Verification items for this drawing (mm, ordinates from the low corner). A direction names the side the tool comes from. Round coordinates to 2 decimals unless told otherwise and drop trailing zeros. Order: outer loops, then holes, each group sorted by start corner. A loop starts at its lowest first (then second) coordinate and runs counter-clockwise, first axis right, second up. Notation, with made-up numbers: M -15,-28 L 42,-28 A27 cw 42,-8 Z; hole C 30.25,36.5 d10. An arc over 180 degrees is marked long. Return JSON: item names as keys, results as strings. Group by question number.
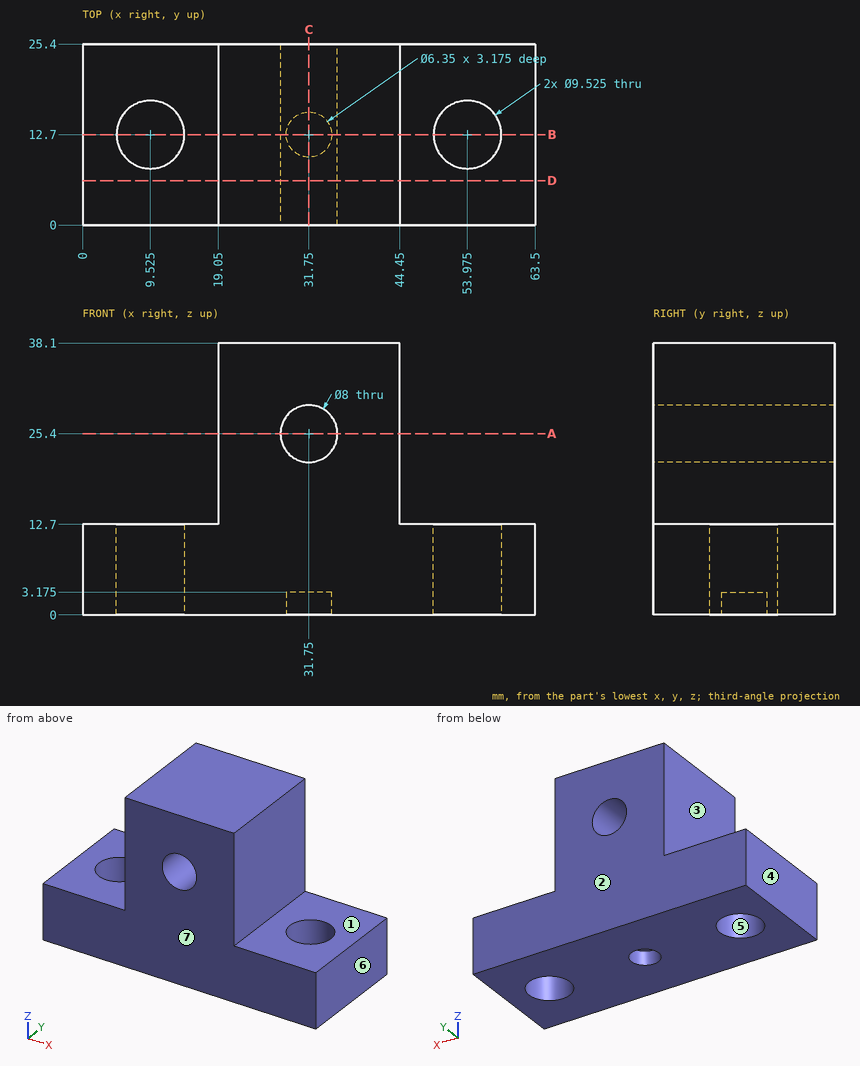
1. Draft check along X on the marked faces 4, 5, 6 and 7. Enter one of: +X half, -X half, draft (parallel to the pull), parting line (faces both ways), or undercut.
2. Cross-section at D-D (y = 6.25). Enter the section's corners in (x, z), plus the area to 3 significant figures.
3. Go/stop test with flat-tipped pins: pin 1 (4 mm diameter, centred on y = 21.5, z = 19.5, fed in from -X); pin 2 (9.5 mm diameter, centred on x = 11.5, y = 17.5, fed in from +Z); pin 3 (5 mm diameter, centred on y = 8, z = 31, fed in from +X). Record where each tip stops, or that it passes through.
4. Cross-section at B-B (y = 12.7). Give the number of separate pieces and of enclosed holes in the cut face, plus the area to 3 significant figures.
5. Thickness scan on line 1 along Z through (x, y) = (31.75, 17); line 2 along Z through (x, y) = (54, 5.25); line 3 along Y through (x, z) = (31.75, 1.55) (3 decimals). Record the ranges inside material, lowest first. Write a range as from..to.
6. Cross-section at C-C (x = 31.75). Enter the section's corners in (y, z) (3 decimals), plus the area to 3 significant figures.
7. Access from +Z, -Z, +X, -X, +Y, -Y to the whole of each face (thin tool, end or side, straight path). Record for the marked faces 1, 2 and 3.
8. Cross-section at A-A (z = 25.4). Enter the section's corners in (x, y), plus the area to 3 significant figures.
Computed:
{
 "1": {"face 4": "-X half", "face 5": "undercut", "face 6": "+X half", "face 7": "draft"},
 "2": {"outline": "M 0,0 L 63.5,0 L 63.5,12.7 L 44.45,12.7 L 44.45,38.1 L 19.05,38.1 L 19.05,12.7 L 0,12.7 Z; hole C 31.75,25.4 d8", "area": "1,400 mm²"},
 "3": {"pin 1": "stops at x = 19.05", "pin 2": "stops at z = 12.7", "pin 3": "stops at x = 44.45"},
 "4": {"separate pieces": "3", "enclosed holes": "1", "area": "1,140 mm²"},
 "5": {"line 1": "z = 0..21.4, 29.4..38.1", "line 2": "z = 0..12.7", "line 3": "y = 0..9.525, 15.875..25.4"},
 "6": {"outline": "M 0,0 L 9.525,0 L 9.525,3.175 L 15.875,3.175 L 15.875,0 L 25.4,0 L 25.4,21.4 L 0,21.4 Z; M 0,29.4 L 25.4,29.4 L 25.4,38.1 L 0,38.1 Z", "area": "744 mm²"},
 "7": {"face 1": "+Z, +X, +Y, -Y", "face 2": "+Z, -Z, +X, -X, +Y", "face 3": "+Z, -X, +Y, -Y"},
 "8": {"outline": "M 19.05,0 L 27.75,0 L 27.75,25.4 L 19.05,25.4 Z; M 35.75,0 L 44.45,0 L 44.45,25.4 L 35.75,25.4 Z", "area": "442 mm²"}
}
